from build123d import *

# Parameters (mm, degrees)
F1_DEPTH = 101
F2_R     = 26.0281777089
F3_DEPTH = 96.7
F5_DEPTH = 4


with BuildPart() as f1:
    # F0 (on Top) → F1 (new body)
    with BuildSketch(Plane.XY):
        with BuildLine():
            ThreePointArc((23.6903417145, -23.8037893118), (30.5111124696, -0.8521403709), (25.3826190605, 22.5358834478))
            ThreePointArc((25.3826190605, 22.5358834478), (0, 32.2655875029), (-25.3826190605, 22.5358834478))
            ThreePointArc((-25.3826190605, 22.5358834478), (-30.337839801, -0.8458126307), (-23.6903417145, -23.8037893118))
            ThreePointArc((-23.6903417145, -23.8037893118), (0, -32.0909383549), (23.6903417145, -23.8037893118))
        make_face()
    extrude(amount=F1_DEPTH)

    # F2 (on face) → F3 (cut)
    with BuildSketch(Plane.XY.offset(101)):
        with Locations((0.9487959906, 0.2371987939)):
            Circle(F2_R)
    extrude(amount=-F3_DEPTH, mode=Mode.SUBTRACT)

    # F4 (on Top) → F5 (join)
    with BuildSketch(Plane.XY):
        with BuildLine():
            ThreePointArc((41.7664500982, -28.0889039008), (35.9824056468, -2.129560913), (44.7880711781, 22.9663135113))
            ThreePointArc((44.7880711781, 22.9663135113), (38.1340229318, 32.8514713703), (29.3426477198, 40.895377501))
            ThreePointArc((29.3426477198, 40.895377501), (-0.5888166123, 35.3352467721), (-30.6889163173, 39.8950284049))
            ThreePointArc((-30.6889163173, 39.8950284049), (-37.0460992048, 34.0735881566), (-42.3167543976, 27.252801203))
            ThreePointArc((-42.3167543976, 27.252801203), (-35.0812809888, 0.4822388969), (-43.0498754281, -26.0793232617))
            ThreePointArc((-43.0498754281, -26.0793232617), (-36.4116539714, -34.750745765), (-28.0593730131, -41.7862951489))
            ThreePointArc((-28.0593730131, -41.7862951489), (-0.8099307183, -34.1616163684), (26.0475538255, -43.0691051203))
            ThreePointArc((26.0475538255, -43.0691051203), (34.7244350449, -36.4367463829), (41.7664500982, -28.0889039008))
        make_face()
    extrude(amount=F5_DEPTH)


solid = f1.part
Geometry: final body of the model. Coordinates: model frame, mm. A direction names the side the tool comes from. Round coordinates to 2 decimals unless told otherwise and drop trailing zeros. Loops run counter-clockwise (first coordinate to the right, second up) from the corner with the lowest first, then second, coordinate; pieces in that order, holes last.
Q1. Section D-D on x = 32.5. Return loops of the section in (y, z).
Q2. Pin query (flat end, axial travel): P1, Ø3, axis at x = -33.5, y = 3.5, coming from the +Z side; P2, Ø1.5, axis at x = 2.5, y = 23.5, coming from the +Z side; P3, Ø12, axis at x = -26, z = 50, coming from the +Y side. Return the tip coordinate at first contact, or that it passes through.
Q3. Pull-direction query (X, two-part tool) for faces 1 (the cylindrical face through (-1.212, -34.154, 1.972)), 2 (the cylindrical face through (0.389, 32.264, 51.821)), 3 (the cylindrical face through (-36.964, 34.162, 1.972)); classes: released by +X, released by -X, zero draft, split by the parting line, or undercut.
Q4. Material intervals for L1, parallel to X at y = 1, z = 59; L2, parallel to Z at x = 28.5, y = 20.5; L3, parallel to X at y = -7, z = 63.5, sorted ascending.
Q5. Section B-B on y = 3.5. Return loops of the section in (x, z), plus the area to 3 significant figures.
Q6. Access query for faces 4 (the flat face through (1, 1, 4.3)), 5 (the cylindrical face through (34.613, -36.542, 1.972)), 6 (the cylindrical face through (30.498, -1.191, 51.821)), 7 (the cylindrical face through (-0.36, -32.09, 51.82)), 8 (the cylindrical face through (-30.35, -0.51, 51.82)). Directions: +Z, -Z, +X, -X, +Y, -Y. A direction counts if a zero-diameter tool reaches every point of the face in a straight line with its end or side. Return the directions, or none.
Q7. Section A-A on x = 1. Return loops of the section in (y, z).
Q8. Section C-C on z = 71. Return loops of the section in (x, y).
Evaluation:
1. outline: (-38.43, 0) - (38.43, 0) - (38.43, 4) - (-38.43, 4) - close
2. P1: stops at z = 4
2. P2: stops at z = 4.3
2. P3: stops at y = 26.57
3. face 1: undercut
3. face 2: split by the parting line
3. face 3: released by -X
4. L1: x = -30.37 to -25.07, 26.97 to 30.54
4. L2: z = 0 to 4
4. L3: x = -29.72 to -24.05, 25.95 to 29.89
5. outline: (-35.13, 0) - (36.65, 0) - (36.65, 4) - (30.47, 4) - (30.47, 101) - (26.77, 101) - (26.77, 4.3) - (-24.87, 4.3) - (-24.87, 101) - (-30.3, 101) - (-30.3, 4) - (-35.13, 4) - close
5. area: 1,190 mm2
6. face 4: +Z
6. face 5: +Z, -Z, +X, -Y
6. face 6: +Z, +X
6. face 7: +Z, -Y
6. face 8: +Z, -X
7. outline: (-34.24, 0) - (35.38, 0) - (35.38, 4) - (32.25, 4) - (32.25, 101) - (26.27, 101) - (26.27, 4.3) - (-25.79, 4.3) - (-25.79, 101) - (-32.08, 101) - (-32.08, 4) - (-34.24, 4) - close
8. outline: (-25.38, 22.54) arc R49.2 ccw to (-23.69, -23.8) arc R38.01 ccw to (23.69, -23.8) arc R47.95 ccw to (25.38, 22.54) arc R37.97 ccw to start; hole circle Ø52.06 at (0.95, 0.24)
